Source: CAD feature listing. Evaluate the final solid. Frame: model axes, mm. A direction names the side the tool comes from. Give positions to 0.01 mm unless a question says otherwise; leave off trailing zeros. Order: outer loops, then holes, each group sorted by start corner. A loop starts at its lowest first (then second) coordinate and runs counter-clockwise, first axis right, second up. Notation, with made-up numbers: M 25,-13.5 L 69,-13.5 A20 ccw 69,13.5 Z; hole C 11.25,-35.75 d1. An arc over 180 degrees is marked long. Answer in a Markdown table with one row per item. Add a question column.
(1) Section query B-B, the plane x = -17.5. Return loops of the section in (y, z), plus the area to 3 significant figures.
(2) Material intervals for line 1 along Y through (x, z) = (-32.5, -23); line 2 along Z through (x, y) = (-49, 42.5); line 3 along X through (y, z) = (65.5, -36), sorted ascending.
(3) Section query A-A, the plane z = -30.5. Count the separate pieces of the cut face and the enclosed holes in it, plus the area to 3 significant figures.
(4) Set-up query: faces 4 (the face through (-13.963, 41, -41)), 5 (the face through (-38.244, 6.261, -18.475)), 6 (the face through (-49.853, 41, -41)), 7 (the face through (-32, 12.7, -22)). Return all of +Z, -Z, +X, -X, +Y, -Y with unobstructed straight access to the full face (end or side cutting, diameter ignored); none if empty.
(5) Section query C-C, the plane x = -40. Return loops of the section in (y, z), plus the area to 3 significant figures.
(6) Pin query (flat end, axial travel): P1, Ø4, axis at y = 37, z = -39, coming from the -X side; P2, Ø12.5, axis at x = -28, z = -27, coming from the +Y side; P3, Ø1, axis at y = 49, z = -36.5, coming from the +X side; P4, Ø1, axis at x = -51, y = 56, coming from the +Z side. Return the tip coordinate at first contact, or that it passes through.
(7) Mould query, pull axis X, two halves, no side actions, for faces 1 (the face through (-23.63, 73.07, -32.05)), 2 (the face through (-12.844, 6.261, -18.475)), 3 (the face through (-24, 49, -21.991)). Classes: pulls with the +X half, pulls with the -X half, needs draft (parallel to the pull), parting line crosses it, or undercut.
(8) Section query D-D, the plane z = -19.5. Return loops of the section in (x, y), plus the area to 3 significant figures.
Autodesk Inventor part; units mm, degrees
ref_plane "YZ Plane" through (0, 0, 0) normal (1, 0, 0) x (0, 1, 0)
ref_plane "XZ Plane" through (0, 0, 0) normal (0, 1, 0) x (-1, 0, 0)
ref_plane "XY Plane" through (0, 0, 0) normal (0, 0, 1) x (1, 0, 0)
sketch "Sketch1" plane through (0, 0, 0) normal (0, 1, 0) x (-1, 0, 0)
  line L0 (6.9046, -9.2909) -> (57.7046, -9.2909)
  line L1 (57.7046, -9.2909) -> (57.7046, -47.3909)
  line L2 (57.7046, -47.3909) -> (6.9046, -47.3909)
  line L3 (6.9046, -47.3909) -> (6.9046, -9.2909)
  point P0 (0, 0)
  dimension "d0" = 50.8
  dimension "d1" = 38.1
extrude "Extrusion1" add sketch "Sketch1" along normal blind 12.7
fillet "Fillet1" radius 6.35 2 edges at (-6.9046, 6.35, -9.2909) (-57.7046, 6.35, -9.2909)
sketch "Sketch2" plane through (0, 12.7, 0) normal (0, 1, 0) x (1, 0, 0)
  point P0 (0, 0)
  point P1 (-19.6046, 21.9909)
  point P2 (-45.0046, 21.9909)
sketch "Sketch3" plane through (0, 12.7, 0) normal (0, 1, 0) x (1, 0, 0)
  line L0 (-6.9046, 47.3909) -> (-6.9046, 15.6409)
  line L1 (-57.7046, 47.3909) -> (-6.9046, 47.3909)
  line L2 (-6.9046, 47.3909) -> (-6.9046, 34.6909)
  line L3 (-6.9046, 34.6909) -> (-57.7046, 34.6909)
  line L4 (-57.7046, 34.6909) -> (-57.7046, 47.3909)
  point P0 (0, 0)
  dimension "d16" = 12.7
extrude "Extrusion2" add sketch "Sketch3" along normal blind 63.5
sketch "Sketch4" plane through (-57.7046, 12.7, -34.6909) normal (0, 0, 1) x (1, 0, 0)
  line L0 (0, 0) -> (6.35, 0)
  arc A0 (43.7412, 12.7) -> (50.8, 0) centre (56.3756, 11.4106) ccw
  line L1 (43.7412, 12.7) -> (43.7412, 44.45)
  line L2 (44.45, 0) -> (50.8, 0)
  arc A1 (0, 0) -> (7.8514, 12.7) centre (-4.8133, 11.7526) ccw
  line L3 (7.8514, 12.7) -> (7.8514, 44.45)
  circle A2 centre (25.7961, 44.45) radius 17.9451
  circle A3 centre (25.7961, 44.45) radius 9.525
  line L4 (0, 0) -> (50.8, 0)
  arc A4 (43.7412, 44.45) -> (7.8514, 44.45) centre (25.7963, 44.45) ccw
  arc A5 (7.8514, 44.45) -> (43.7412, 44.45) centre (25.7963, 44.45) ccw
  line L5 (0, 0) -> (0, 63.5)
  line L6 (0, -12.7) -> (0, 63.5)
  line L7 (0, 63.5) -> (50.8, 63.5)
  line L8 (50.8, 63.5) -> (50.8, 0)
  line L9 (50.8, -12.7) -> (50.8, 63.5)
  point P0 (57.7046, -12.7)
extrude "Extrusion3" cut sketch "Sketch4" against normal blind 25.4 contours L5 L7 L8 A0 L1 A2 L3 A1
extrude "Extrusion4" cut sketch "Sketch4" against normal blind 25.4 contours A3
extrude "Extrusion5" add sketch "Sketch4" along normal blind 12.7 contours A2
hole "Hole2" at (-19.6046, 12.7, -21.9909) at (-45.0046, 12.7, -21.9909) direction (0, -1, 0) diameter 15.24 end through all
properties part number "7.1 Part 5"
Values follow:
| question | item | result |
|---|---|---|
| 1 | outline | M 0,-47.39 L 67.85,-47.39 L 67.85,-21.99 L 46.45,-21.99 L 46.45,-34.69 L 12.7,-34.69 L 12.7,-29.31 L 0,-29.31 Z; M 0,-14.67 L 12.7,-14.67 L 12.7,-9.29 L 0,-9.29 Z |
| 1 | area | 1,270 mm² |
| 2 | line 1 | y = 0 to 12.7, 39.21 to 47.64, 66.66 to 75.09 |
| 2 | line 2 | z = -47.39 to -34.69 |
| 2 | line 3 | x = -47.79 to -36.49, -27.33 to -16.02 |
| 3 | separate pieces | 2 |
| 3 | enclosed holes | 1 |
| 3 | area | 1,370 mm² |
| 4 | face 4 | +Z, -Z, +X, +Y |
| 4 | face 5 | -Y |
| 4 | face 6 | +Z, -Z, -X, +Y |
| 4 | face 7 | +Z, +X, -X |
| 5 | outline | M 0,-47.39 L 52.12,-47.39 L 52.12,-21.99 L 41.13,-21.99 L 41.13,-34.69 L 12.7,-34.69 L 12.7,-27.74 L 0,-27.74 Z; M 0,-16.24 L 12.7,-16.24 L 12.7,-9.29 L 0,-9.29 Z; M 62.18,-47.39 L 73.17,-47.39 L 73.17,-21.99 L 62.18,-21.99 Z |
| 5 | area | 1,260 mm² |
| 6 | P1 | stops at x = -49.85 |
| 6 | P2 | stops at y = 75.1 |
| 6 | P3 | stops at x = -13.96 |
| 6 | P4 | passes through |
| 7 | face 1 | parting line crosses it |
| 7 | face 2 | undercut |
| 7 | face 3 | needs draft |
| 8 | outline | M -57.7,0 L -52.21,0 L -52.21,12.7 L -57.7,12.7 Z; M -37.8,0 L -26.81,0 L -26.81,12.7 L -37.8,12.7 Z; M -12.4,0 L -6.9,0 L -6.9,12.7 L -12.4,12.7 Z |
| 8 | area | 279 mm² |
